Part model, mm, in its own coordinate system. A direction names the side the tool comes from. Give positions to 0.01 mm unless a question says otherwise; leave off trailing zeros. Order: outer loops, then holes, each group sorted by start corner. A loop starts at its lowest first (then second) coordinate and runs counter-clockwise, first axis right, second up. Notation, with made-up numbers: (69, 79.5) - (124, 79.5) arc R19 ccw to (124, 112.5) - close; hole circle Ø9 at (86, 87). An arc over 180 degrees is marked (long way). One line per item, written item: value.
```python
from build123d import *

# Parameters (mm, degrees)
BOSS_EXTRUDE1_DEPTH = 2
SKETCH1_4_R         = 1.75
BOSS_EXTRUDE2_DEPTH = 4.5


with BuildPart() as part:
    # Sketch1 → Boss-Extrude1 (new body)
    with BuildSketch(Plane.XY):
        with BuildLine():
            ThreePointArc((4, 0), (0, 4), (-4, 0))
            Line((-4, 0), (-4, -16))
            ThreePointArc((-4, -16), (0, -20), (4, -16))
            Line((4, -16), (4, 0))
        make_face()
    extrude(amount=-BOSS_EXTRUDE1_DEPTH)

    # Sketch1<4> → Boss-Extrude2 (add)
    with BuildSketch(Plane.XY):
        Circle(SKETCH1_4_R)
        with Locations((0, -16)):
            Circle(SKETCH1_4_R)
    extrude(amount=BOSS_EXTRUDE2_DEPTH)


solid = part.part
```
1) Which spindle directions (+Z, -Z, +X, -X, +Y, -Y) get a long thin tool onto all of the face, cutting with end or side? Do faces 4 (the flat face through (4, -8, -1)), 5 (the cylindrical face through (1.617, -0.67, 2.218)). Say none if no direction does.
Outcome:
face 4: +Z, -Z, +X, +Y, -Y
face 5: +Z
2) Drill centre lines: line 1 along Z through (x, y) = (-2, -2.75); line 2 along Y through (x, z) = (-0.5, 3.75); line 3 along Y through (x, z) = (1.5, 1.25). Where is each one in solid material? Low to high. Write a range as from..to.
Outcome:
line 1: z = -2..0
line 2: y = -17.68..-14.32, -1.68..1.68
line 3: y = -16.9..-15.1, -0.9..0.9
3) Mould opens along Y. For faces 1 (the flat face through (0, 0, 4.5)), 2 (the cylindrical face through (-0.228, -14.265, 2.218)), 3 (the cylindrical face through (0, -20, -1)) say: released by +Y, released by -Y, zero draft, split by the parting line, or undercut.
Outcome:
face 1: zero draft
face 2: undercut
face 3: released by -Y
4) Cut at C-C, the plane y = -11.25. Give the cut face in (x, z), then the cut area to 3 significant figures.
Outcome:
outline: (-4, -2) - (4, -2) - (4, 0) - (-4, 0) - close
area: 16.0 mm^2
5) Cut at A-A, the plane x = 0. Give the cut face in (y, z), then the cut area to 3 significant figures.
Outcome:
outline: (-20, -2) - (4, -2) - (4, 0) - (1.75, 0) - (1.75, 4.5) - (-1.75, 4.5) - (-1.75, 0) - (-14.25, 0) - (-14.25, 4.5) - (-17.75, 4.5) - (-17.75, 0) - (-20, 0) - close
area: 79.5 mm^2
6) Cut at B-B, the plane z = 2.75. Give the cut face in (x, y), then the cut area to 3 significant figures.
Outcome:
outline: circle Ø3.5 at (0, -16); circle Ø3.5 at (0, 0)
area: 19.2 mm^2
7) Pin check, flat tips, straight feed: pin 1 (2 mm diameter, centred on x = -1.5, y = -7, fed in from +Z); pin 2 (1.5 mm diameter, centred on x = -1, z = -0.5, fed in from +Y). Stop position of each tip, or through.
Outcome:
pin 1: stops at z = 0
pin 2: stops at y = 3.99
8) Cut at D-D, the plane y = -15. Give the cut face in (x, z), then the cut area to 3 significant figures.
Outcome:
outline: (-4, -2) - (4, -2) - (4, 0) - (1.44, 0) - (1.44, 4.5) - (-1.44, 4.5) - (-1.44, 0) - (-4, 0) - close
area: 28.9 mm^2
